Study the drawing (mm; zero at the part's minimum x, y, z) and answer. Coordinates: 2 decimals unless noted, no trailing zeros. Loops run counter-clockwise (first coordinate to the right, second up) from the corner with the lowest first, then second, coordinate; pieces in that order, holes last. Notation, with made-up numbers: (21, 51.25) -> (57, 51.25) arc R23 cw to (57, 68.25) -> close; hole circle Ø11 at (32.5, 13.5). An arc over 180 degrees is marked (long way). One line per question, with ' | ' between items.
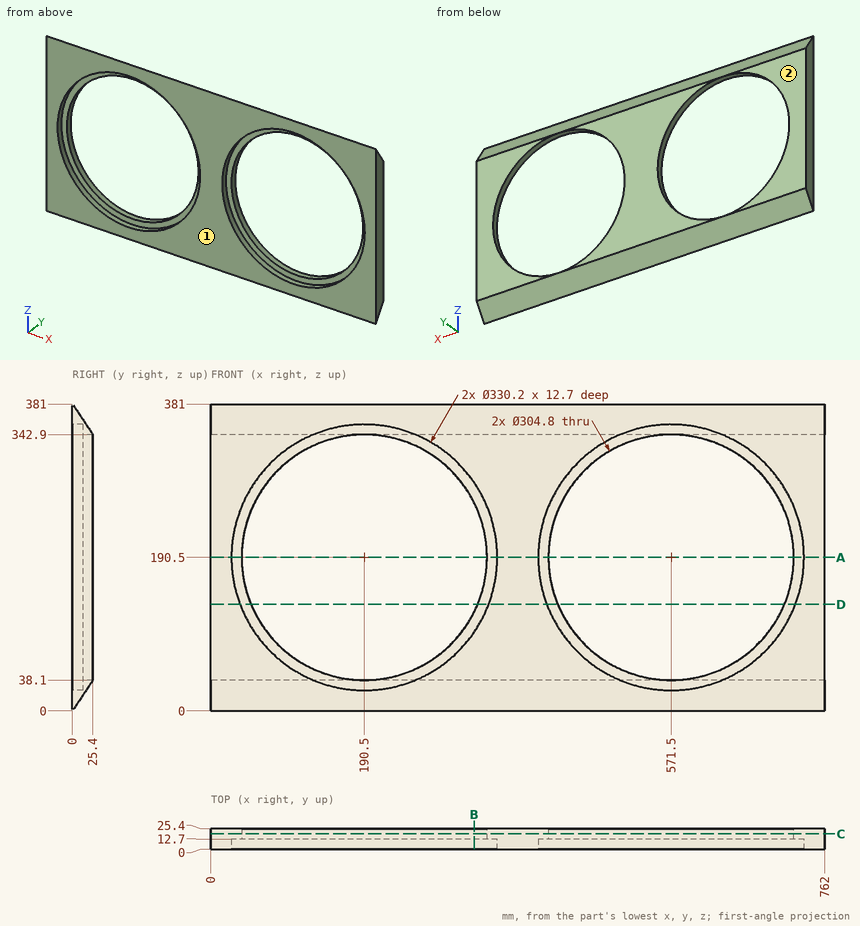
1) Find the intervals of material crossed by line 1 along X through (y, z) = (20.75, 190.5); line 2 along X through (y, z) = (12.25, 169); line 3 along Z through (x, y) = (571.5, 18.25) (3 decimals), in increasing order.
Check values:
line 1: x = 0 to 38.1, 342.9 to 419.1, 723.9 to 762 | line 2: x = 0 to 26.81, 354.19 to 407.81, 735.19 to 762 | line 3: z = 27.375 to 38.1, 342.9 to 353.625
2) Find section A-A (z = 190.5). Write down the section's boundary in (x, y), plus the area to 3 significant figures.
Check values:
outline: (0, 0) -> (25.4, 0) -> (25.4, 12.7) -> (38.1, 12.7) -> (38.1, 25.4) -> (0, 25.4) -> close; (342.9, 12.7) -> (355.6, 12.7) -> (355.6, 0) -> (406.4, 0) -> (406.4, 12.7) -> (419.1, 12.7) -> (419.1, 25.4) -> (342.9, 25.4) -> close; (723.9, 12.7) -> (736.6, 12.7) -> (736.6, 0) -> (762, 0) -> (762, 25.4) -> (723.9, 25.4) -> close | area: 3,230 mm^2
3) Flat-ended cylindrical pins translate along their axes: pin 1 (12 mm diameter, centred on x = 95, y = 14.5, fed in from -Z); pin 2 (3 mm diameter, centred on x = 265.5, y = 20, fed in from +Z); pin 3 (5 mm diameter, centred on x = 383, y = 16, fed in from +Z). Find the tip coordinate at first contact, or state that the pin passes through.
Check values:
pin 1: stops at z = 12.75 | pin 2: stops at z = 353.25 | pin 3: stops at z = 360.75
4) Find section C-C (y = 19). Write down the section's boundary in (x, z), plus the area to 3 significant figures.
Check values:
outline: (0, 28.5) -> (762, 28.5) -> (762, 352.5) -> (0, 352.5) -> close; hole circle Ø304.8 at (190.5, 190.5); hole circle Ø304.8 at (571.5, 190.5) | area: 101,000 mm^2
5) The mould has two halves that part along Y. Classify the marked faces 1 and 2: released by +Y, released by -Y, zero draft, split by the parting line, or undercut.
Check values:
face 1: released by -Y | face 2: released by +Y
6) Find section D-D (z = 132). Write down the section's boundary in (x, y).
Check values:
outline: (0, 0) -> (36.11, 0) -> (36.11, 12.7) -> (49.78, 12.7) -> (49.78, 25.4) -> (0, 25.4) -> close; (331.22, 12.7) -> (344.89, 12.7) -> (344.89, 0) -> (417.11, 0) -> (417.11, 12.7) -> (430.78, 12.7) -> (430.78, 25.4) -> (331.22, 25.4) -> close; (712.22, 12.7) -> (725.89, 12.7) -> (725.89, 0) -> (762, 0) -> (762, 25.4) -> (712.22, 25.4) -> close
7) Find section B-B (x = 327). Write down the section's boundary in (y, z), plus the area to 3 significant figures.
Check values:
outline: (0, 0) -> (25.4, 38.1) -> (25.4, 122.72) -> (12.7, 122.72) -> (12.7, 97.63) -> (0, 97.63) -> close; (0, 283.37) -> (12.7, 283.37) -> (12.7, 258.28) -> (25.4, 258.28) -> (25.4, 342.9) -> (0, 381) -> close | area: 4,630 mm^2
